The listing builds one solid part. Answer for the finished solid, in the listing's coordinates (mm). Face numbers are marked on the shaded views. Coordinates: 2 decimals unless noted, no trailing zeros. Write each loop counter-clockwise with the first axis right and the second up, starting at its lowest first coordinate (ties: lowest second). Pieces come first, ordered by that corner, then holes.
from build123d import *

# Parameters (mm, degrees)
F0_W     = 114.572242
F0_H     = 99.697284
F1_DEPTH = 25.4
F2_R     = 12.7
F2_R_2   = 6.35
F2_R_3   = 15.24
F2_R_4   = 25.4
F3_DEPTH = 25.4
F4_R     = 2.54


with BuildPart() as f1:
    # F0 (on Front) → F1 (new body)
    with BuildSketch(Plane.XZ):
        with Locations((4e-06, -1.034044)):
            Rectangle(F0_W, F0_H)
    extrude(amount=F1_DEPTH)

    # F2 (on Front) → F3 (cut)
    with BuildSketch(Plane.XZ):
        with Locations((-29.891482, 28.83641)):
            Circle(F2_R)
        with Locations((29.859781, 26.308896)):
            Circle(F2_R_2)
        with Locations((-28.831949, -25.76586)):
            Circle(F2_R_3)
        with Locations((28.062282, -21.096375)):
            Circle(F2_R_4)
    extrude(amount=F3_DEPTH, mode=Mode.SUBTRACT)

    # F4
    f4_edges = [f1.edges().sort_by_distance(p)[0] for p in [
        (4e-06, -25.4, 48.814598),
        (-57.286117, -12.7, 48.814598),
        (4e-06, 0, 48.814598),
        (57.286125, -12.7, 48.814598),
        (57.286125, -25.4, -1.034044),
        (57.286125, 0, -1.034044),
        (-57.286117, -25.4, -1.034044),
        (4e-06, -25.4, -50.882686),
        (57.286125, -12.7, -50.882686),
        (4e-06, 0, -50.882686),
        (-57.286117, -12.7, -50.882686),
        (-57.286117, 0, -1.034044),
    ]]
    fillet(f4_edges, radius=F4_R)


solid = f1.part
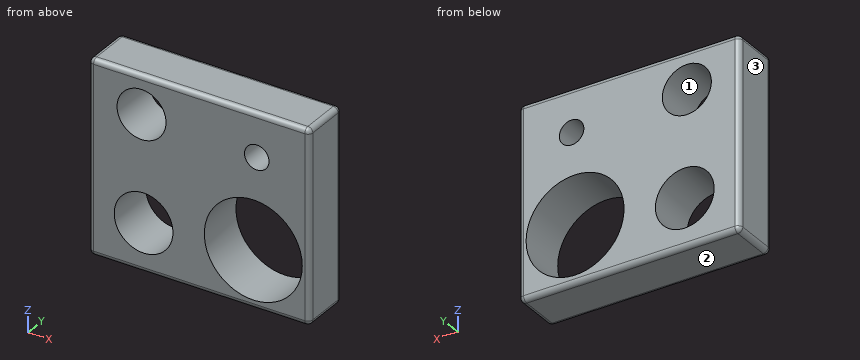
1. Section A-A on x = -28 is taken. Give the vertices of the cut face in (y, z), then the cut area to 3 significant figures.
Results found:
outline: (-25.4, -48.34) arc R2.54 ccw to (-22.86, -50.88) - (-2.54, -50.88) arc R2.54 ccw to (0, -48.34) - (0, -40.98) - (-25.4, -40.98) - close; (-25.4, -10.55) - (0, -10.55) - (0, 16.28) - (-25.4, 16.28) - close; (-25.4, 41.39) - (0, 41.39) - (0, 46.27) arc R2.54 ccw to (-2.54, 48.81) - (-22.86, 48.81) arc R2.54 ccw to (-25.4, 46.27) - close
area: 1,120 mm2
2. Find the intervals of material crossed by L1, parallel to Z at x = 24.5, y = -13.5; L2, parallel to X at y = -6.75, z = -18.5; L3, parallel to Z at x = 28.5, y = -13.5, in increasing order.
Results found:
L1: z = -50.88 to -46.25, 4.05 to 22.9, 29.71 to 48.81
L2: x = -57.29 to -42.23, -15.44 to 2.8, 53.33 to 57.29
L3: z = -50.88 to -46.49, 4.3 to 20.11, 32.51 to 48.81
3. Section B-B on z = 35 is taken. Give the vertices of the cut face in (x, y), then the cut area to 3 significant figures.
Results found:
outline: (-57.29, -22.86) arc R2.54 ccw to (-54.75, -25.4) - (-41, -25.4) - (-41, 0) - (-54.75, 0) arc R2.54 ccw to (-57.29, -2.54) - close; (-18.79, -25.4) - (54.75, -25.4) arc R2.54 ccw to (57.29, -22.86) - (57.29, -2.54) arc R2.54 ccw to (54.75, 0) - (-18.79, 0) - close
area: 2,340 mm2
4. Section C-C on x = 45.5 is taken. Give the vertices of the cut face in (y, z), then the cut area to 3 significant figures.
Results found:
outline: (-25.4, -48.34) arc R2.54 ccw to (-22.86, -50.88) - (-2.54, -50.88) arc R2.54 ccw to (0, -48.34) - (0, -39.56) - (-25.4, -39.56) - close; (-25.4, -2.63) - (0, -2.63) - (0, 46.27) arc R2.54 ccw to (-2.54, 48.81) - (-22.86, 48.81) arc R2.54 ccw to (-25.4, 46.27) - close
area: 1,590 mm2
5. Section D-D on y = -4.25 is taken. Give the vertices of the cut face in (x, z), then the cut area to 3 significant figures.
Results found:
outline: (-57.29, -48.34) arc R2.54 ccw to (-54.75, -50.88) - (54.75, -50.88) arc R2.54 ccw to (57.29, -48.34) - (57.29, 46.27) arc R2.54 ccw to (54.75, 48.81) - (-54.75, 48.81) arc R2.54 ccw to (-57.29, 46.27) - close; hole circle Ø30.48 at (-28.83, -25.77); hole circle Ø25.4 at (-29.89, 28.84); hole circle Ø50.8 at (28.06, -21.1); hole circle Ø12.7 at (29.86, 26.31)
area: 8,030 mm2
6. A flat-ended cylindrical pin translates along its axis: P1, Ø18.5, axis at x = -28.83, z = -25.77, coming from the +Y side. Find the tip coordinate at first contact, or state that the pin passes through.
Results found:
P1: passes through
7. For a pull along X with two mould halves and no side action, classify the marked faces 1, 2 and 3 as pulls with the +X half, pulls with the -X half, needs draft (parallel to the pull), parting line crosses it, or undercut.
Results found:
face 1: undercut
face 2: needs draft
face 3: pulls with the -X half
